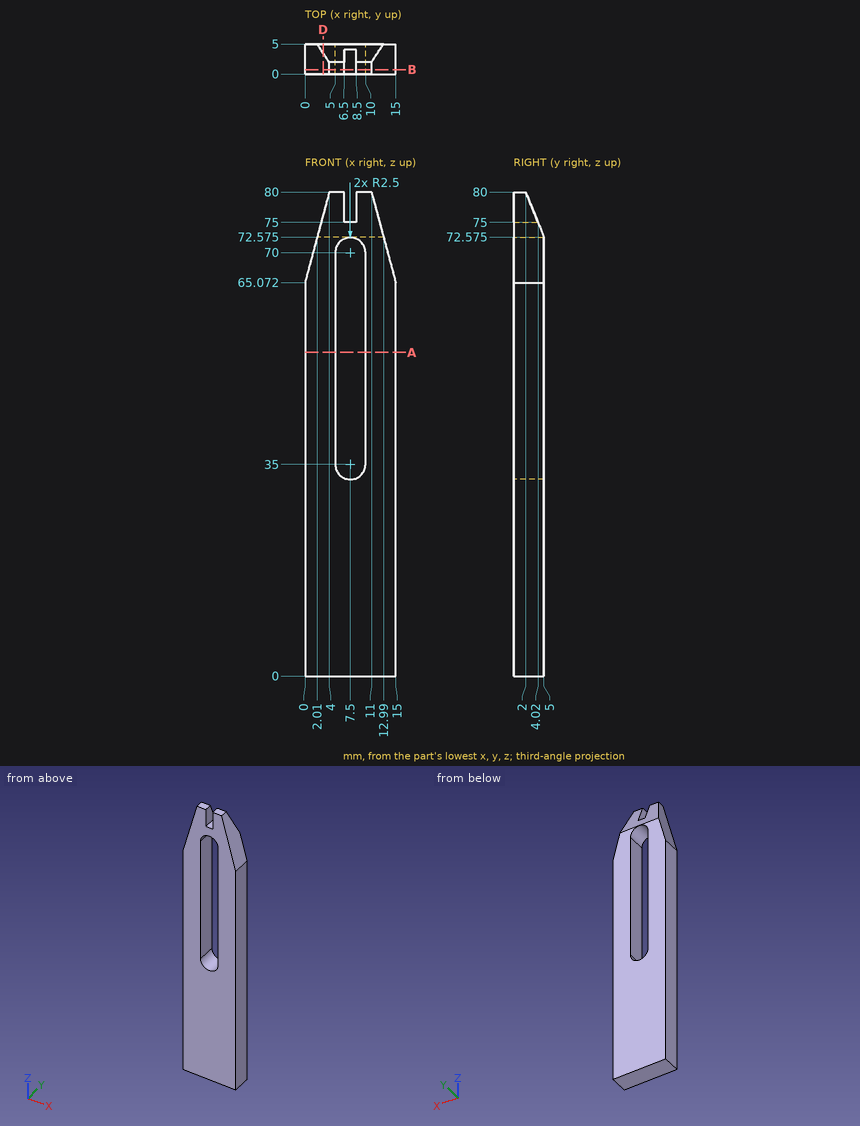
Drawing for the job (mm, zero at the part's lowest x, y, z). Round coordinates to 2 decimals unless told otherwise and drop trailing zeros. Order: outer loops, then holes, each group sorted by start corner. A loop starts at its lowest first (then second) coordinate and runs counter-clockwise, first axis right, second up. Notation, with made-up numbers: (-15.5, 52) -> (0.5, 52) arc R20 cw to (0.5, 79) -> close; hole circle Ø4 at (-5, 29). An arc over 180 degrees is marked (long way). Put each result on its own line as item: value.
Q1. Band-saw the part on B-B (y = 0.75). Give the cut face in (x, z).
From the geometry:
outline: (0, 0) -> (15, 0) -> (15, 65.07) -> (11, 80) -> (8.5, 80) -> (8.5, 75) -> (6.5, 75) -> (6.5, 80) -> (4, 80) -> (0, 65.07) -> close; hole (5, 35) arc R2.5 ccw to (10, 35) -> (10, 70) arc R2.5 ccw to (5, 70) -> close
Q2. Wall check: line 1 (X direction, y = 3.2, z = 36); line 2 (Z direction, x = 7.75, y = 3.45); line 3 (Z direction, x = 6.75, y = 2.5) (1 decimal). Give the ranges that are in metal, low to high. Write a range as [from, to].
From the geometry:
line 1: x = [0, 5], [10, 15]
line 2: z = [0, 32.51], [72.49, 75]
line 3: z = [0, 32.6], [72.4, 75]
Q3. Band-saw the part on A-A (z = 53.5). Give the cut face in (x, y), and give its area (3 significant figures).
From the geometry:
outline: (0, 0) -> (5, 0) -> (5, 5) -> (0, 5) -> close; (10, 0) -> (15, 0) -> (15, 5) -> (10, 5) -> close
area: 50.0 mm2
Q4. Pin check, flat tips, straight feed: pin 1 Ø1.2 at (y, z) = (1.5, 77.5) entering from +X; pin 2 Ø1 at (x, y) = (5.5, 4) entering from +Z (1 decimal). Stop position of each tip, or through.
From the geometry:
pin 1: stops at x = 11.83
pin 2: stops at z = 76.3
Q5. Band-saw the part on D-D (x = 3). Give the cut face in (y, z) (1 decimal).
From the geometry:
outline: (0, 0) -> (5, 0) -> (5, 72.6) -> (3.5, 76.3) -> (0, 76.3) -> close
